For this review, take the finished solid that the model builds, in its own axes (mm). A direction names the side the tool comes from. Coordinates: 2 decimals unless noted, no trailing zeros. Write each loop counter-clockwise with the first axis right and the second up, starting at its lowest first coordinate (ties: lowest second). Pieces come first, ordered by that corner, then holes. Notation, with made-up numbers: M -9,6.25 L 43,6.25 A7 ccw 43,14.25 Z; hole C 75.25,66 d5. An arc over 180 degrees is marked long. One line per question, with ' | ' between items.
Autodesk Inventor part; units mm, degrees
ref_plane "YZ Plane" through (0, 0, 0) normal (1, 0, 0) x (0, 1, 0)
ref_plane "XZ Plane" through (0, 0, 0) normal (0, 1, 0) x (-1, 0, 0)
ref_plane "XY Plane" through (0, 0, 0) normal (0, 0, 1) x (1, 0, 0)
sketch "Sketch1" plane through (0, 0, 0) normal (0, 1, 0) x (-1, 0, 0)
  line L0 (0, 0) -> (-35, 0)
  line L1 (-35, 0) -> (-35, -35)
  line L2 (-35, -35) -> (0, -35)
  line L3 (0, -35) -> (0, 0)
  dimension "d0" = 35
  dimension "d1" = 35
extrude "Extrusion1" add sketch "Sketch1" along normal blind 110
sketch "Sketch2" plane through (0, 110, 0) normal (0, 1, 0) x (1, 0, 0)
  line L0 (0, 35) -> (0, 0) construction
  line L1 (0, 0) -> (35, 0) construction
  line L2 (0, 35) -> (35, 0) construction
  circle A0 centre (17.5, 17.5) radius 11.75
  dimension "d4" = 23.5
extrude "Extrusion2" cut sketch "Sketch2" against normal blind 50
sketch "Sketch3" plane through (0, 0, 0) normal (0, -1, 0) x (1, 0, 0)
  line L0 (35, -35) -> (0, -35) construction
  line L1 (35, -35) -> (0, 0) construction
  circle A0 centre (17.5, -17.5) radius 11.75
  dimension "d7" = 23.5
extrude "Extrusion3" cut sketch "Sketch3" against normal blind 50
sketch "Sketch4" plane through (0, 0, 0) normal (0, 0, 1) x (1, 0, 0)
  circle A0 centre (17.5, 90) radius 1.75
  line L0 (0, 110) -> (35, 110)
  circle A1 centre (17.5, 20) radius 1.75
  line L1 (0, 0) -> (35, 0)
  line L2 (0, 0) -> (0, 110)
  line L3 (35, 0) -> (35, 110)
  dimension "d10" = 3.5
  dimension "d11" = 20
  dimension "d12" = 3.5
  dimension "d13" = 20
  dimension "d24" = 35
  dimension "d25" = 17.5
  dimension "d26" = 17.5
extrude "Extrusion4" cut sketch "Sketch4" against normal blind 36 contours A0 | A1
sketch "Sketch5" plane through (0, 0, -35) normal (-1, 0, 0) x (0, 0, 1)
  circle A0 centre (17.5, 90) radius 1.75
  circle A1 centre (17.5, 20) radius 1.75
  line L0 (0, 110) -> (35, 110)
  line L1 (0, 0) -> (35, 0)
  line L2 (0, 0) -> (0, 110)
  line L3 (35, 0) -> (35, 110)
  dimension "d16" = 3.5
  dimension "d17" = 3.5
  dimension "d18" = 20
  dimension "d19" = 20
  dimension "d27" = 35
  dimension "d28" = 17.5
  dimension "d29" = 17.5
extrude "Extrusion5" cut sketch "Sketch5" against normal blind 36 contours A0 | A1
fillet "Fillet1" radius 10 4 edges at (35, 55, 0) (35, 55, -35) (0, 55, -35) (0, 55, 0)
equation "\"d25\" = 0.5 * d24"
equation "\"d26\" = 0.5 * d24"
equation "\"d28\" = 0.5 * d27"
equation "\"d29\" = 0.5 * d27"
properties part number "Rod_Joint_v2"
1) We need section A-A on z = -17.5. State the section outline as (x, y) points.
Responses:
outline: M 0,0 L 5.75,0 L 5.75,18.25 L 0,18.25 Z; M 0,21.75 L 5.75,21.75 L 5.75,50 L 29.25,50 L 29.25,21.75 L 35,21.75 L 35,88.25 L 29.25,88.25 L 29.25,60 L 5.75,60 L 5.75,88.25 L 0,88.25 Z; M 0,91.75 L 5.75,91.75 L 5.75,110 L 0,110 Z; M 29.25,0 L 35,0 L 35,18.25 L 29.25,18.25 Z; M 29.25,91.75 L 35,91.75 L 35,110 L 29.25,110 Z
2) We need section C-C on x = 17.5. State the section outline as (y, z) points, then the cut area to 3 significant figures.
Responses:
outline: M 0,-35 L 18.25,-35 L 18.25,-29.25 L 0,-29.25 Z; M 0,-5.75 L 18.25,-5.75 L 18.25,0 L 0,0 Z; M 21.75,-35 L 88.25,-35 L 88.25,-29.25 L 60,-29.25 L 60,-5.75 L 88.25,-5.75 L 88.25,0 L 21.75,0 L 21.75,-5.75 L 50,-5.75 L 50,-29.25 L 21.75,-29.25 Z; M 91.75,-35 L 110,-35 L 110,-29.25 L 91.75,-29.25 Z; M 91.75,-5.75 L 110,-5.75 L 110,0 L 91.75,0 Z | area: 1,420 mm^2
3) Insertion check: pin 1 Ø5.5 at (x, y) = (17.5, 90) entering from -Z; pin 2 Ø14 at (x, z) = (17.5, -17.5) entering from +Y; pin 3 Ø1 at (x, y) = (28, 74) entering from +Z; pin 4 Ø7 at (x, z) = (15.5, -12.5) entering from -Y. Each pin has a flat end and moves straight along its axis. Give the tip position at first contact, or say it passes through.
Responses:
pin 1: z = -35 | pin 2: y = 60 | pin 3: z = -0.32 | pin 4: y = 50
4) The part is to be moulded in two halves that separate along X. For faces 4 (the flat face through (17, 60, -18)), 5 (the cylindrical face through (2.9, 88.29, -17.88)), 6 (the cylindrical face through (31.99, 55.77, -2.85)), say which applies: +X half, -X half, draft (parallel to the pull), parting line (faces both ways), or undercut.
Responses:
face 4: undercut | face 5: draft | face 6: +X half
5) We need section B-B on y = 90. State the section outline as (x, z) points, then the cut area to 3 significant figures.
Responses:
outline: M 0,-25 A10 ccw 10,-35 L 15.75,-35 L 15.75,-29.12 A11.75 cw 5.88,-19.25 L 0,-19.25 Z; M 0,-15.75 L 5.88,-15.75 A11.75 cw 15.75,-5.88 L 15.75,0 L 10,0 A10 ccw 0,-10 Z; M 19.25,-35 L 25,-35 A10 ccw 35,-25 L 35,-19.25 L 29.12,-19.25 A11.75 cw 19.25,-29.12 Z; M 19.25,-5.88 A11.75 cw 29.12,-15.75 L 35,-15.75 L 35,-10 A10 ccw 25,0 L 19.25,0 Z | area: 624 mm^2
6) To check wall thickness, follow line 1 along Y through (x, z) = (1.2, -17.5); line 2 along Z through (x, y) = (17, 72); line 3 along Y through (x, z) = (14, -26). State the ranges of each line that lie inside material, in increasing order. Write a range as [from, to].
Responses:
line 1: [0, 18.25], [21.75, 88.25], [91.75, 110] | line 2: [-35, -29.24], [-5.76, 0] | line 3: [50, 60]
7) We need section D-D on y = 30. State the section outline as (x, z) points.
Responses:
outline: M 0,-25 A10 ccw 10,-35 L 25,-35 A10 ccw 35,-25 L 35,-10 A10 ccw 25,0 L 10,0 A10 ccw 0,-10 Z; hole C 17.5,-17.5 d23.5
8) Machinability: for faces 1 (the flat face through (29.4, 0, -17.3)), 2 (the cylindrical face through (28.707, 85.35, -21.029)), 3 (the cylindrical face through (28.707, 24.65, -13.971)), which of the approach directions +Z, -Z, +X, -X, +Y, -Y give a long, thin tool a straight path to every point of the face, cutting with its end or side? Answer none if there is none.
Responses:
face 1: +Z, -Z, +X, -X, -Y | face 2: +Y | face 3: -Y
